```python
from build123d import *

# Parameters (mm, degrees)
SKETCH1_R           = 1.9
BOSS_EXTRUDE1_DEPTH = 13
CHAMFER1_SIZE       = 0.5
SKETCH4_W           = 1
SKETCH4_H           = 0.407466182
SKETCH7_W           = 1
SKETCH7_H           = 0.36313202


with BuildPart() as part:
    # Sketch1 → Boss-Extrude1 (new body)
    with BuildSketch(Plane.XY):
        with Locations(Location((0, 0, 0), (0, 0, 180))):
            Circle(SKETCH1_R)
    extrude(amount=BOSS_EXTRUDE1_DEPTH)

    # Chamfer1
    chamfer1_edges = [part.edges().sort_by_distance(p)[0] for p in [
        (1.9, 0, 13),
    ]]
    chamfer(chamfer1_edges, length=CHAMFER1_SIZE)

    # Sketch4 → Cut-Revolve4 (revolve, cut)
    with BuildSketch(Plane(origin=(0, 0, 0), x_dir=(0, 0, -1), z_dir=(1, 0, 0)), mode=Mode.PRIVATE) as cut_revolve4_sk:
        with Locations((-10.5, 1.9)):
            Rectangle(SKETCH4_W, SKETCH4_H)
    revolve(cut_revolve4_sk.sketch.rotate(Axis((0, 0, 14.953462275), (0, 0, -1)), 270), axis=Axis((0, 0, 14.953462275), (0, 0, -1)), mode=Mode.SUBTRACT)

    # Sketch7 → Cut-Revolve7 (revolve, cut)
    with BuildSketch(Plane(origin=(0, 0, 0), x_dir=(0, 0, -1), z_dir=(1, 0, 0)), mode=Mode.PRIVATE) as cut_revolve7_sk:
        with Locations((-6.5, 1.9)):
            Rectangle(SKETCH7_W, SKETCH7_H)
    revolve(cut_revolve7_sk.sketch.rotate(Axis((0, 0, 14.336983713), (0, 0, -1)), 270), axis=Axis((0, 0, 14.336983713), (0, 0, -1)), mode=Mode.SUBTRACT)


solid = part.part
```
Input: part model. Units: mm. Frame: model coordinates. A direction names the side the tool comes from. Round coordinates to 2 decimals unless told otherwise and drop trailing zeros. Loops run counter-clockwise (first coordinate to the right, second up) from the corner with the lowest first, then second, coordinate; pieces in that order, holes last. Notation, with made-up numbers: M 79.5,16 L 129.5,16 A16 ccw 129.5,39 Z; hole C 19,78.5 d9. An arc over 180 degrees is marked long. Answer in a Markdown table with one row per item. Add a question column.
1. Contact query for a flat-ended pin moving along its axis: pin 1 (1 mm diameter, centred on y = -1, z = 4, fed in from +X). Output: stop coordinate, or through.
2. Section C-C (z = 10.25). Output: boundary loops of the cut face in (x, y).
3. Set-up query: faces 1 (the face through (0.22, 1.68, 10.49)), 2 (the face through (0, 0, 0)). Return all of +Z, -Z, +X, -X, +Y, -Y with unobstructed straight access to the full face (end or side cutting, diameter ignored); none if empty.
4. Ray query, probe 1 along X at (y, z) = (0.1, 1.25); probe 2 along Z at (x, y) = (-0.9, -1.4). Return the intervals inside material, ascending.
5. Section A-A (x = 0). Output: boundary loops of the cut face in (y, z), and give its area (3 significant figures).
6. Section D-D (z = 1.5). Output: boundary loops of the cut face in (x, y), and give its area (3 significant figures).
Values follow:
| question | item | result |
|---|---|---|
| 1 | pin 1 | x = 1.83 |
| 2 | outline | C 0,0 d3.39 |
| 3 | face 1 | none |
| 3 | face 2 | -Z, +X, -X, +Y, -Y |
| 4 | probe 1 | -1.9 to 1.9 |
| 4 | probe 2 | 0 to 12.74 |
| 5 | outline | M -1.9,0 L 1.9,0 L 1.9,6 L 1.72,6 L 1.72,7 L 1.9,7 L 1.9,10 L 1.7,10 L 1.7,11 L 1.9,11 L 1.9,12.5 L 1.4,13 L -1.4,13 L -1.9,12.5 L -1.9,11 L -1.7,11 L -1.7,10 L -1.9,10 L -1.9,7 L -1.72,7 L -1.72,6 L -1.9,6 Z |
| 5 | area | 48.4 mm^2 |
| 6 | outline | C 0,0 d3.8 |
| 6 | area | 11.3 mm^2 |
